from build123d import *

# Parameters (mm, degrees)
SKETCH1_R           = 11.43
BOSS_EXTRUDE1_DEPTH = 152.4
SKETCH2_R           = 10.133203601
CUT_EXTRUDE1_DEPTH  = 149.86
CUT_EXTRUDE2_DEPTH  = 12.7


with BuildPart() as part:
    # Sketch1 → Boss-Extrude1 (new body)
    with BuildSketch(Plane.XY):
        with Locations(Location((0, 0, 0), (0, 0, 180))):
            Circle(SKETCH1_R)
    extrude(amount=BOSS_EXTRUDE1_DEPTH)

    # Sketch2 → Cut-Extrude1 (cut)
    with BuildSketch(Plane.XY.offset(152.4)):
        Circle(SKETCH2_R)
    extrude(amount=-CUT_EXTRUDE1_DEPTH, mode=Mode.SUBTRACT)

    # Sketch3 → Cut-Extrude2 (cut)
    with BuildSketch(Plane(origin=(0, 0, 0), x_dir=(0, 0, -1), z_dir=(1, 0, 0))):
        with BuildLine():
            Line((-10.671040116, -5.903350135), (-140.211040116, -5.903350135))
            ThreePointArc((-140.211040116, -5.903350135), (-146.114390251, 0), (-140.211040116, 5.903350135))
            Line((-140.211040116, 5.903350135), (-10.671040116, 5.903350135))
            ThreePointArc((-10.671040116, 5.903350135), (-4.767689981, 0), (-10.671040116, -5.903350135))
        make_face()
    extrude(amount=-CUT_EXTRUDE2_DEPTH, mode=Mode.SUBTRACT)


solid = part.part
The model under review builds one solid part; all positions refer to its coordinate system, in mm. A direction names the side the tool comes from. Give positions to 0.01 mm unless a question says otherwise; leave off trailing zeros. Order: outer loops, then holes, each group sorted by start corner. A loop starts at its lowest first (then second) coordinate and runs counter-clockwise, first axis right, second up. Notation, with made-up numbers: M 85,75.25 L 96,75.25 A20 ccw 96,107.25 Z; hole C 66.25,31 d7. An arc over 180 degrees is marked long. One line per question, with ' | ' between items. Start each with the question number.
1) Wall thickness on L1, parallel to Y at x = 0, z = 116.5; L2, parallel to Z at x = -7.5, y = -6.75; L3, parallel to Y at x = -4, z = 131: over which ranges is each line inside the solid? List them lowest first. Write a range as from..to.
2) Consider section C-C, the plane y = -4.5. Give the boundary of the cut face in (x, z), then the cut area to 3 significant figures.
3) Consider section D-D, the plane z = 95.5. Give the boundary of the cut face in (x, y), then the cut area to 3 significant figures.
4) Clearance check with flat-ended pins moving along their axes: P1, Ø6, axis at x = -7.5, z = 53, coming from the +Y side; P2, Ø1, axis at x = 3.5, y = -7.5, coming from the +Z side; P3, Ø12, axis at y = -1.5, z = 33, coming from the -X side. State where each tip first meets the part, or that it passes through.
5) For faces 1 (the face through (-10.52, 0.13, 4.77)), 2 (the face through (0, 0, 2.54)), 3 (the face through (7, 8, 152.4)), list the 3-axis set-ups (+Z, -Z, +X, -X, +Y, -Y) from which the entire face can be reached by the end or side of a thin tool; tool diameter is ignored.
6) Mouldability with a two-part tool opening along X and no side actions: class faces 4 (the face through (11.42, -0.5, 75.13)), 5 (the face through (0, 0, 0)), 6 (the face through (9.665, 3.044, 78.519)) as pulls with the +X half, pulls with the -X half, needs draft (parallel to the pull), parting line crosses it, or undercut.
7) Consider section A-A, the plane y = 3.5. Give the boundary of the cut face in (x, z), then the cut area to 3 significant figures.
8) Consider section B-B, the plane x = 0. Give the boundary of the cut face in (y, z), then the cut area to 3 significant figures.
Found:
1) L1: y = -11.43..-10.13, 10.13..11.43 | L2: z = 0..2.54 | L3: y = -10.71..-9.31, 9.31..10.71
2) outline: M -10.51,0 L 10.51,0 L 10.51,152.4 L 9.08,152.4 L 9.08,2.54 L -9.08,2.54 L -9.08,6.85 L -10.51,6.85 Z; M -10.51,144.03 L -9.08,144.03 L -9.08,152.4 L -10.51,152.4 Z | area: 285 mm²
3) outline: M -9.79,-5.9 A11.43 ccw long -9.79,5.9 L -8.24,5.9 A10.13 cw long -8.24,-5.9 Z | area: 71.6 mm²
4) P1: stops at y = 10.51 | P2: stops at z = 2.54 | P3: stops at x = -9.79
5) face 1: -X | face 2: +Z | face 3: +Z, +X, -X, +Y, -Y
6) face 4: parting line crosses it | face 5: needs draft | face 6: undercut
7) outline: M -10.88,0 L 10.88,0 L 10.88,152.4 L 9.51,152.4 L 9.51,2.54 L -9.51,2.54 L -9.51,5.92 L -10.88,5.92 Z; M -10.88,144.96 L -9.51,144.96 L -9.51,152.4 L -10.88,152.4 Z | area: 276 mm²
8) outline: M -11.43,0 L 11.43,0 L 11.43,152.4 L 10.13,152.4 L 10.13,2.54 L -10.13,2.54 L -10.13,152.4 L -11.43,152.4 Z | area: 447 mm²
